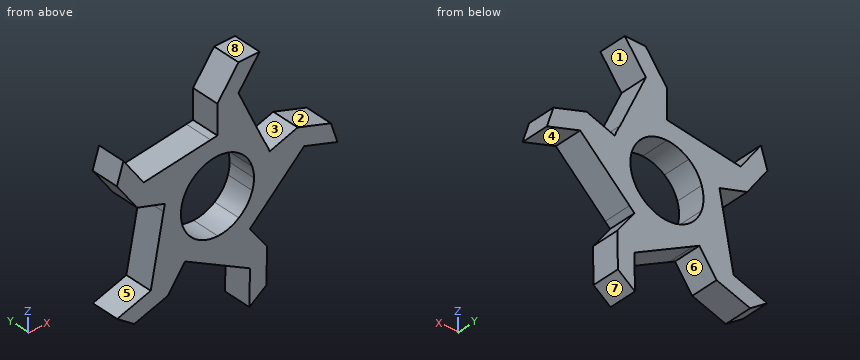
```python
from build123d import *

# Parameters (mm, degrees)
F1_DEPTH = 5


with BuildPart() as f1:
    # F0 (on Front) → F1 (new body)
    with BuildSketch(Plane.XZ):
        with BuildLine():
            ThreePointArc((6.2807772336, 2.0407482309), (6.5226938013, 1.0330932071), (6.604, 0))
            ThreePointArc((6.604, 0), (6.5294502373, -0.9894925964), (6.3074840707, -1.9566452661))
            Line((6.3074840707, -1.9566452661), (9.8738155336, -0.7978739305))
            ThreePointArc((9.8738155336, -0.7978739305), (9.897950613, -0.3992613959), (9.906, 0))
            ThreePointArc((9.906, 0), (9.7840407019, 1.5496398107), (9.4211658504, 3.0611223463))
            Line((9.4211658504, 3.0611223463), (6.2807772336, 2.0407482309))
        make_face()
        with BuildLine():
            ThreePointArc((3.81, 5.3941371877), (5.3166954651, 3.9173416154), (6.2807772336, 2.0407482309))
            Line((6.2807772336, 2.0407482309), (9.4211658504, 3.0611223463))
            Line((9.4211658504, 3.0611223463), (8.4486177468, 5.1720106505))
            ThreePointArc((8.4486177468, 5.1720106505), (6.4430274028, 7.5243759799), (3.81, 9.144))
            Line((3.81, 9.144), (3.81, 5.3941371877))
        make_face()
        with BuildLine():
            Line((9.8738155336, -0.7978739305), (6.3074840707, -1.9566452661))
            ThreePointArc((6.3074840707, -1.9566452661), (5.3685625225, -3.8459527353), (3.8817338061, -5.3427482309))
            Line((3.8817338061, -5.3427482309), (5.8226007092, -8.0141223463))
            ThreePointArc((5.8226007092, -8.0141223463), (6.3048332162, -7.6405440981), (6.763157516, -7.2379925679))
            ThreePointArc((6.763157516, -7.2379925679), (8.9199775829, -4.3084609689), (9.8738155336, -0.7978739305))
        make_face()
        with BuildLine():
            Line((14.4941013083, 4.7094189943), (9.4211658504, 3.0611223463))
            ThreePointArc((9.4211658504, 3.0611223463), (9.7840407019, 1.5496398107), (9.906, 0))
            ThreePointArc((9.906, 0), (9.897950613, -0.3992613959), (9.8738155336, -0.7978739305))
            Line((9.8738155336, -0.7978739305), (15.6714560569, 1.0858936672))
            Line((15.6714560569, 1.0858936672), (14.4941013083, 4.7094189943))
        make_face()
        with BuildLine():
            Line((8.4486177468, 5.1720106505), (9.4211658504, 3.0611223463))
            ThreePointArc((9.4211658504, 3.0611223463), (8.9970136051, 4.1451878352), (8.4486177468, 5.1720106505))
        make_face()
        with BuildLine():
            Line((15.6714560569, 1.0858936672), (9.8738155336, -0.7978739305))
            ThreePointArc((9.8738155336, -0.7978739305), (8.9199775829, -4.3084609689), (6.763157516, -7.2379925679))
            Line((6.763157516, -7.2379925679), (15.6714560569, 1.0858936672))
        make_face()
        with BuildLine():
            ThreePointArc((-3.9527745736, 5.2904053881), (-2.0826640172, 6.2670029992), (0, 6.604))
            Line((0, 6.604), (0, 9.906))
            ThreePointArc((0, 9.906), (-0.6097179629, 9.8872180114), (-1.2171238492, 9.8309432679))
            ThreePointArc((-1.2171238492, 9.8309432679), (-4.6839635346, 8.7286494721), (-7.5191060364, 6.4491767236))
            Line((-7.5191060364, 6.4491767236), (-3.9527745736, 5.2904053881))
        make_face()
        with BuildLine():
            Line((3.81, 15.24), (3.81, 9.144))
            ThreePointArc((3.81, 9.144), (6.4430274028, 7.5243759799), (8.4486177468, 5.1720106505))
            Line((8.4486177468, 5.1720106505), (3.81, 15.24))
        make_face()
        with BuildLine():
            ThreePointArc((0, 9.906), (1.9427264347, 9.7136321734), (3.81, 9.144))
            Line((3.81, 9.144), (3.81, 15.24))
            Line((3.81, 15.24), (0, 15.24))
            Line((0, 15.24), (0, 9.9816298047))
            Line((0, 9.9816298047), (0, 9.906))
        make_face()
        Polygon((20.5028231597, 2.6556999986), (14.4941013083, 4.7094189943), (15.6714560569, 1.0858936672), (21.6801779083, -0.9678253285), align=None)
        with BuildLine():
            Line((2.2923535984, -9.6371132078), (0.0882395392, -6.6034104661))
            ThreePointArc((0.0882395392, -6.6034104661), (-1.9987413555, -6.2942711249), (-3.8817338061, -5.3427482309))
            Line((-3.8817338061, -5.3427482309), (-5.8226007092, -8.0141223463))
            ThreePointArc((-5.8226007092, -8.0141223463), (-5.3182886736, -8.3573106669), (-4.793809454, -8.6688076988))
            ThreePointArc((-4.793809454, -8.6688076988), (-1.3411652542, -9.8147904593), (2.2923535984, -9.6371132078))
        make_face()
        with BuildLine():
            Line((5.8670547931, -8.0753081436), (5.8226007092, -8.0141223463))
            ThreePointArc((5.8226007092, -8.0141223463), (4.1378310366, -9.0003994529), (2.2923535984, -9.6371132078))
            Line((2.2923535984, -9.6371132078), (5.8754924964, -14.5688808055))
            Line((5.8754924964, -14.5688808055), (8.9578472449, -12.3294189943))
            Line((8.9578472449, -12.3294189943), (5.8670547931, -8.0753081436))
        make_face()
        with BuildLine():
            ThreePointArc((6.763157516, -7.2379925679), (6.3048332162, -7.6405440981), (5.8226007092, -8.0141223463))
            Line((5.8226007092, -8.0141223463), (5.8670547931, -8.0753081436))
            Line((5.8670547931, -8.0753081436), (6.763157516, -7.2379925679))
        make_face()
        with BuildLine():
            ThreePointArc((-1.2171238492, 9.8309432679), (-0.6097179629, 9.8872180114), (0, 9.906))
            Line((0, 9.906), (0, 9.9816298047))
            Line((0, 9.9816298047), (-1.2171238492, 9.8309432679))
        make_face()
        Polygon((3.81, 20.32), (3.81, 15.24), (7.62, 20.32), align=None)
        Polygon((0, 15.24), (3.81, 15.24), (3.81, 20.32), align=None)
        with BuildLine():
            Line((5.8754924964, -14.5688808055), (2.2923535984, -9.6371132078))
            ThreePointArc((2.2923535984, -9.6371132078), (-1.3411652542, -9.8147904593), (-4.793809454, -8.6688076988))
            Line((-4.793809454, -8.6688076988), (5.8754924964, -14.5688808055))
        make_face()
        with BuildLine():
            ThreePointArc((-6.2529490364, -2.1244868436), (-6.6038526149, -0.0441207543), (-6.2807772336, 2.0407482309))
            Line((-6.2807772336, 2.0407482309), (-9.4211658504, 3.0611223463))
            ThreePointArc((-9.4211658504, 3.0611223463), (-9.5917163846, 2.47544194), (-9.7258946926, 1.8803745449))
            ThreePointArc((-9.7258946926, 1.8803745449), (-9.7488632535, -1.7574132312), (-8.4570630955, -5.1581895853))
            Line((-8.4570630955, -5.1581895853), (-6.2529490364, -2.1244868436))
        make_face()
        with BuildLine():
            Line((-13.3167465598, 8.3329443214), (-7.5191060364, 6.4491767236))
            ThreePointArc((-7.5191060364, 6.4491767236), (-4.6839635346, 8.7286494721), (-1.2171238492, 9.8309432679))
            Line((-1.2171238492, 9.8309432679), (-13.3167465598, 8.3329443214))
        make_face()
        with BuildLine():
            ThreePointArc((-9.4211658504, 3.0611223463), (-8.6378776917, 4.8493200538), (-7.5191060364, 6.4491767236))
            Line((-7.5191060364, 6.4491767236), (-13.3167465598, 8.3329443214))
            Line((-13.3167465598, 8.3329443214), (-14.4941013083, 4.7094189943))
            Line((-14.4941013083, 4.7094189943), (-9.493094069, 3.0844932412))
            Line((-9.493094069, 3.0844932412), (-9.4211658504, 3.0611223463))
        make_face()
        with BuildLine():
            Line((-5.8670547931, -8.0753081436), (-5.8226007092, -8.0141223463))
            ThreePointArc((-5.8226007092, -8.0141223463), (-7.2812284388, -6.7165875578), (-8.4570630955, -5.1581895853))
            Line((-8.4570630955, -5.1581895853), (-12.0402019935, -10.089957183))
            Line((-12.0402019935, -10.089957183), (-8.9578472449, -12.3294189943))
            Line((-8.9578472449, -12.3294189943), (-5.8670547931, -8.0753081436))
        make_face()
        with BuildLine():
            ThreePointArc((-4.793809454, -8.6688076988), (-5.3182886736, -8.3573106669), (-5.8226007092, -8.0141223463))
            Line((-5.8226007092, -8.0141223463), (-5.8670547931, -8.0753081436))
            Line((-5.8670547931, -8.0753081436), (-4.793809454, -8.6688076988))
        make_face()
        Polygon((8.9578472449, -12.3294189943), (5.8754924964, -14.5688808055), (5.7790868294, -20.9181489482), (8.861441578, -18.6786871369), align=None)
        with BuildLine():
            ThreePointArc((-9.7258946926, 1.8803745449), (-9.5917163846, 2.47544194), (-9.4211658504, 3.0611223463))
            Line((-9.4211658504, 3.0611223463), (-9.493094069, 3.0844932412))
            Line((-9.493094069, 3.0844932412), (-9.7258946926, 1.8803745449))
        make_face()
        Polygon((-14.4941013083, 4.7094189943), (-13.3167465598, 8.3329443214), (-16.970758914, 13.5262759799), (-18.1481136625, 9.9027506528), align=None)
        with BuildLine():
            Line((-12.0402019935, -10.089957183), (-8.4570630955, -5.1581895853))
            ThreePointArc((-8.4570630955, -5.1581895853), (-9.7488632535, -1.7574132312), (-9.7258946926, 1.8803745449))
            Line((-9.7258946926, 1.8803745449), (-12.0402019935, -10.089957183))
        make_face()
        Polygon((-8.9578472449, -12.3294189943), (-12.0402019935, -10.089957183), (-18.1085058237, -11.9603017032), (-15.0261510752, -14.1997635145), align=None)
        with BuildLine():
            Line((-5.8226007092, -8.0141223463), (-3.8817338061, -5.3427482309))
            ThreePointArc((-3.8817338061, -5.3427482309), (-5.3166954651, -3.9173416154), (-6.2529490364, -2.1244868436))
            Line((-6.2529490364, -2.1244868436), (-8.4570630955, -5.1581895853))
            ThreePointArc((-8.4570630955, -5.1581895853), (-7.2812284388, -6.7165875578), (-5.8226007092, -8.0141223463))
        make_face()
        with BuildLine():
            Line((5.8226007092, -8.0141223463), (3.8817338061, -5.3427482309))
            ThreePointArc((3.8817338061, -5.3427482309), (2.0826640172, -6.2670029992), (0.0882395392, -6.6034104661))
            Line((0.0882395392, -6.6034104661), (2.2923535984, -9.6371132078))
            ThreePointArc((2.2923535984, -9.6371132078), (4.1378310366, -9.0003994529), (5.8226007092, -8.0141223463))
        make_face()
        with BuildLine():
            ThreePointArc((-6.2807772336, 2.0407482309), (-5.3685625225, 3.8459527353), (-3.9527745736, 5.2904053881))
            Line((-3.9527745736, 5.2904053881), (-7.5191060364, 6.4491767236))
            ThreePointArc((-7.5191060364, 6.4491767236), (-8.6378776917, 4.8493200538), (-9.4211658504, 3.0611223463))
            Line((-9.4211658504, 3.0611223463), (-6.2807772336, 2.0407482309))
        make_face()
        with BuildLine():
            ThreePointArc((0, 6.604), (1.9987413555, 6.2942711249), (3.81, 5.3941371877))
            Line((3.81, 5.3941371877), (3.81, 9.144))
            ThreePointArc((3.81, 9.144), (1.9427264347, 9.7136321734), (0, 9.906))
            Line((0, 9.906), (0, 6.604))
        make_face()
    extrude(amount=F1_DEPTH)


solid = f1.part
```
Could you check a few things on this model? Use its own coordinates, in mm. Face numbers are marked on the shaded views. A direction names the side the tool comes from. Round coordinates to 2 decimals unless told otherwise and drop trailing zeros. Loops run counter-clockwise (first coordinate to the right, second up) from the corner with the lowest first, then second, coordinate; pieces in that order, holes last. Notation, with made-up numbers: (-1.5, 19.25) - (43.5, 19.25) arc R26 cw to (43.5, 52.25) - close; hole circle Ø9 at (-22.5, 31). An arc over 180 degrees is marked (long way). Answer in a Markdown table with one row per item. Add a question column.
(1) I need wall thicknesses on line 1 along Z through (x, y) = (4, -4.4); line 2 along Z through (x, y) = (7.5, -2.3); line 3 along Z through (x, y) = (2.5, -4.4). Which ranges of each line are inside material? Lowest first, please.
(2) If we mould it in two halves opening along X, with no side actions, what happens to the marked faces 6, 7 and 8? For each: pulls with the +X half, pulls with the -X half, needs draft (parallel to the pull), parting line crosses it, or undercut.
(3) If we section it at A-A (x = 3): Please give me the cut outline in (y, z), plus the area to 3 significant figures.
(4) If we section it at B-B (z = -18): Please give me the cut outline in (x, y).
(5) I'm going to push flat-ended pins straight in: pin 1 (2 mm diameter, centred on x = -12, y = -3.5, fed in from -Z); pin 2 (1 mm diameter, centred on y = -1, z = -2, fed in from -X); pin 3 (1 mm diameter, centred on y = -2.5, z = 6, fed in from -X). Where does each tip first touch, or does it pass through?
(6) For the marked faces 1, 2, 3, 4 and 5, which set-ups out of +Z, -Z, +X, -X, +Y, -Y let a thin tool reach every point of the face, with its end or its side?
(7) If we section it at C-C (x = 15): Please give me the cut outline in (y, z).
Model answer:
| question | item | result |
|---|---|---|
| 1 | line 1 | z = -13.53 to -5.25, 5.25 to 14.83, 15.49 to 20.32 |
| 1 | line 2 | z = -19.67 to -10.32, -6.55 to 7.23, 20.16 to 20.32 |
| 1 | line 3 | z = -12.7 to -6.11, 6.11 to 18.57 |
| 2 | face 6 | undercut |
| 2 | face 7 | pulls with the +X half |
| 2 | face 8 | needs draft |
| 3 | outline | (-5, -12.98) - (0, -12.98) - (0, -5.88) - (-5, -5.88) - close; (-5, 5.88) - (0, 5.88) - (0, 19.24) - (-5, 19.24) - close |
| 3 | area | 102 mm² |
| 4 | outline | (5.82, -5) - (8.87, -5) - (8.87, 0) - (5.82, 0) - close |
| 5 | pin 1 | stops at z = -13.58 |
| 5 | pin 2 | stops at x = -10.57 |
| 5 | pin 3 | stops at x = -15.75 |
| 6 | face 1 | +X, +Y, -Y |
| 6 | face 2 | +Z, +X, +Y, -Y |
| 6 | face 3 | +Z, +Y, -Y |
| 6 | face 4 | -Z, +Y, -Y |
| 6 | face 5 | -X, +Y, -Y |
| 7 | outline | (-5, 0.46) - (0, 0.46) - (0, 4.54) - (-5, 4.54) - close |
